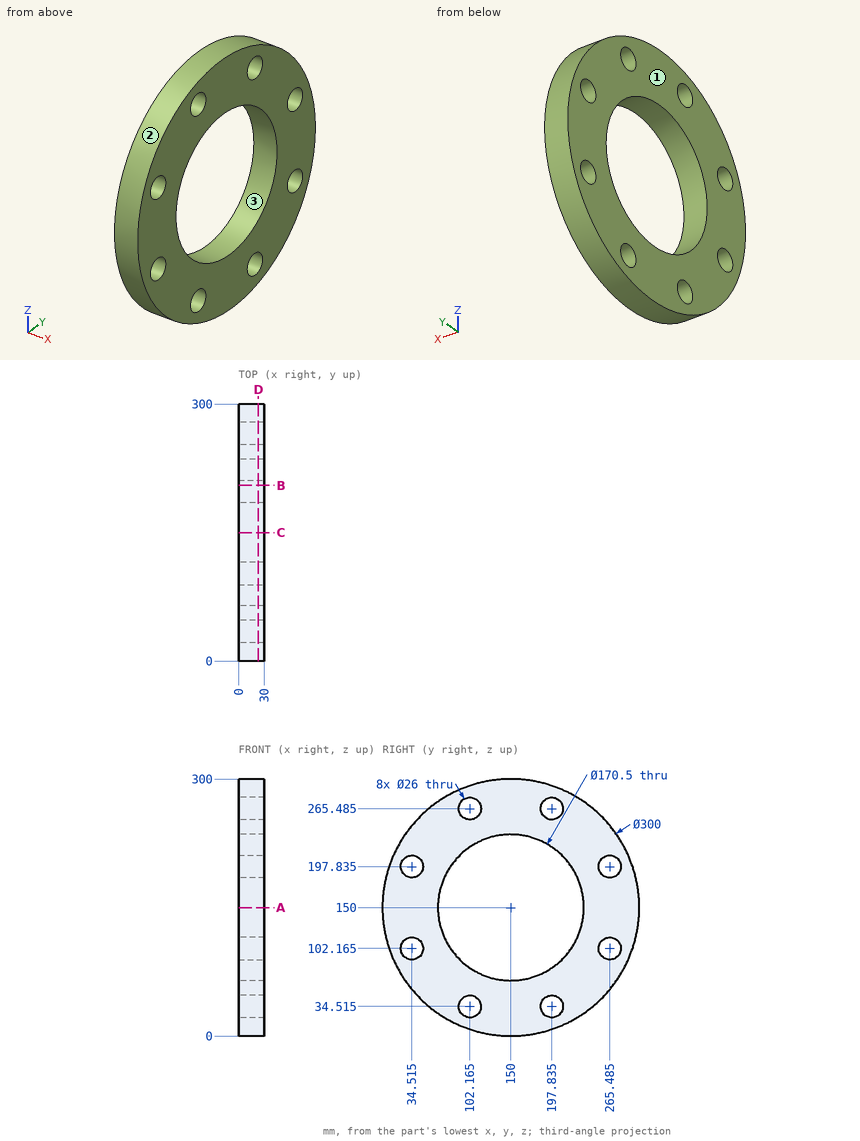
The drawing under review shows one solid part. Ordinate dimensions are in mm from its lowest x, y, z. Round coordinates to 2 decimals unless told otherwise and drop trailing zeros. Loops run counter-clockwise (first coordinate to the right, second up) from the corner with the lowest first, then second, coordinate; pieces in that order, holes last. Notation, with made-up numbers: (12, 43.25) - (44, 43.25) arc R25 ccw to (44, 76.25) - close; hole circle Ø2 at (-3, 21.25). An arc over 180 degrees is marked (long way). Put each result on its own line as item: value. Start each with the question number.
1. Insertion check: P1, Ø2, axis at x = 14.5, y = 35, coming from the +Z side; P2, Ø1.5, axis at x = 6, y = 78.5, coming from the -Z side; P3, Ø2, axis at x = 6.5, y = 189, coming from the +Z side; P4, Ø21, axis at y = 102.16, z = 265.48, coming from the -X side. Each pin has a flat end and moves straight along its axis. Give the tip position at first contact, or say it passes through.
2. Consider section B-B on y = 205. State the section outline as (x, z) points (1 decimal).
3. Mouldability with a two-part tool opening along Z and no side actions: class the marked faces 1, 2 and 3 as +Z half, -Z half, draft (parallel to the pull), parting line (faces both ways), or undercut.
4. Consider section D-D on x = 23. State how many separate pieces and enclosed holes the cut face has, plus the area to 3 significant figures.
5. For probe 1 along Y at (x, z) = (19.25, 202) (1 decimal); probe 2 along Z at (x, y) = (15.5, 150); probe 3 along Y at (x, z) = (5, 46.5) (1 decimal), list the stretches that pass through material, from the lowest coordinate up. Write a range as [from, to].
6. Consider section A-A on z = 150. State the section outline as (x, y) points, plus the area to 4 significant figures.
Result sheet:
1. P1: z = 247.49
1. P2: z = 17.73
1. P3: z = 295.11
1. P4: through
2. outline: (0, 10.4) - (30, 10.4) - (30, 23.7) - (0, 23.7) - close; (0, 45.4) - (30, 45.4) - (30, 84.9) - (0, 84.9) - close; (0, 215.1) - (30, 215.1) - (30, 254.6) - (0, 254.6) - close; (0, 276.3) - (30, 276.3) - (30, 289.6) - (0, 289.6) - close
3. face 1: draft
3. face 2: parting line
3. face 3: undercut
4. separate pieces: 1
4. enclosed holes: 9
4. area: 43,600 mm^2
5. probe 1: [9.3, 22.2], [46.8, 82.4], [217.6, 253.2], [277.8, 290.7]
5. probe 2: [0, 64.75], [235.25, 300]
5. probe 3: [41.4, 97.1], [107.2, 192.8], [202.9, 258.6]
6. outline: (0, 0) - (30, 0) - (30, 64.75) - (0, 64.75) - close; (0, 235.25) - (30, 235.25) - (30, 300) - (0, 300) - close
6. area: 3,885 mm^2
